Source: three-view drawing plus pictorial views. Frame: mm from the lowest corner of the part. A direction names the side the tool comes from. Give positions to 0.01 mm unless a question says otherwise; leave off trailing zeros. Loops run counter-clockwise (first coordinate to the right, second up) from the corner with the lowest first, then second, coordinate; pieces in that order, holes last. Notation, with made-up numbers: M 66,61 L 87,61 A18 cw 87,81 Z; hole C -25.75,56 d7. An arc over 180 degrees is marked long. Answer as a JSON object with one key per item and string values. Group by question number.
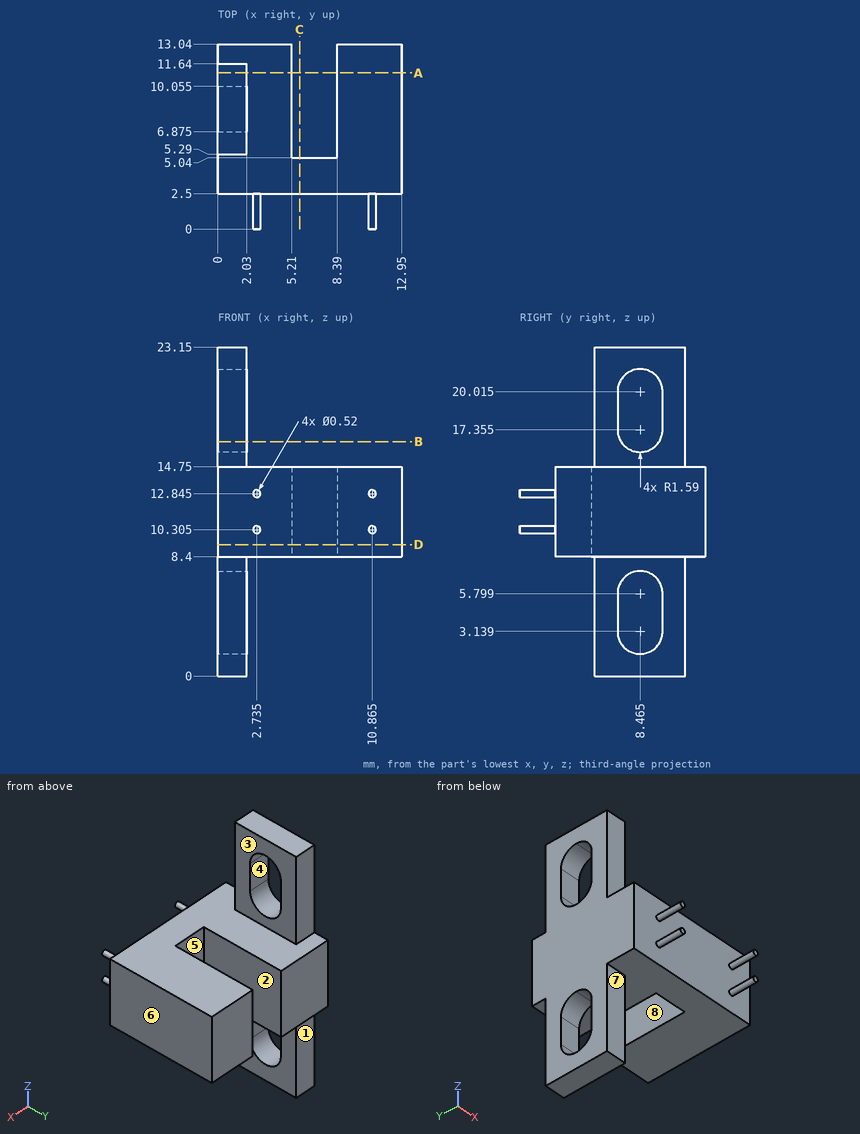
1. Section B-B (z = 16.5). Output: boundary loops of the cut face in (x, y).
2. Mould query, pull axis X, two halves, no side actions, for the marked faces 5, 6, 7 and 8. Classes: pulls with the +X half, pulls with the -X half, needs draft (parallel to the pull), parting line crosses it, or undercut.
3. First-contact query: P1, Ø2, axis at x = 0.5, z = 5, coming from the +Y side; P2, Ø0.6, axis at x = 0.5, z = 18.5, coming from the -Y side; P3, Ø1, axis at x = 9.5, y = 7, coming from the +Z side; P4, Ø3, axis at y = 8, z = 12, coming from the -X side. Flat tips, straight axial feed; report the tip coordinate or a pass-through.
4. Reachability of the marked faces 1, 2, 3 and 4 from +Z, -Z, +X, -X, +Y, -Y: full face, straight path, thin tool, end or side. Return the list, or none.
5. Section C-C (x = 5.75). Output: boundary loops of the cut face in (y, z), then the cut area to 3 significant figures.
6. Section A-A (y = 11). Output: boundary loops of the cut face in (x, z).
7. Section D-D (z = 9.25). Output: boundary loops of the cut face in (x, y).
8. Material intervals for L1, parallel to X at y = 11, z = 8.5; L2, parallel to Z at x = 11.25, y = 8.5; L3, parallel to X at y = 6.75, z = 18.5, sorted ascending.
Geometry results:
{
 "1": {"outline": "M 0,5.29 L 2.03,5.29 L 2.03,7.12 L 0,7.12 Z; M 0,9.81 L 2.03,9.81 L 2.03,11.64 L 0,11.64 Z"},
 "2": {"face 5": "undercut", "face 6": "pulls with the +X half", "face 7": "needs draft", "face 8": "undercut"},
 "3": {"P1": "y = 11.64", "P2": "y = 5.29", "P3": "z = 14.75", "P4": "x = 0"},
 "4": {"face 1": "-Z, +X, -X, +Y", "face 2": "+Z, -Z, +Y", "face 3": "+Z, +X, +Y, -Y", "face 4": "+X, -X"},
 "5": {"outline": "M 2.5,8.4 L 5.04,8.4 L 5.04,14.75 L 2.5,14.75 Z", "area": "16.1 mm2"},
 "6": {"outline": "M 0,0 L 2.03,0 L 2.03,8.4 L 5.21,8.4 L 5.21,14.75 L 2.03,14.75 L 2.03,23.15 L 0,23.15 Z; M 8.39,8.4 L 12.95,8.4 L 12.95,14.75 L 8.39,14.75 Z"},
 "7": {"outline": "M 0,2.5 L 12.95,2.5 L 12.95,13.04 L 8.39,13.04 L 8.39,5.04 L 5.21,5.04 L 5.21,13.04 L 0,13.04 Z"},
 "8": {"L1": "0 to 5.21, 8.39 to 12.95", "L2": "8.4 to 14.75", "L3": "0 to 2.03"}
}
